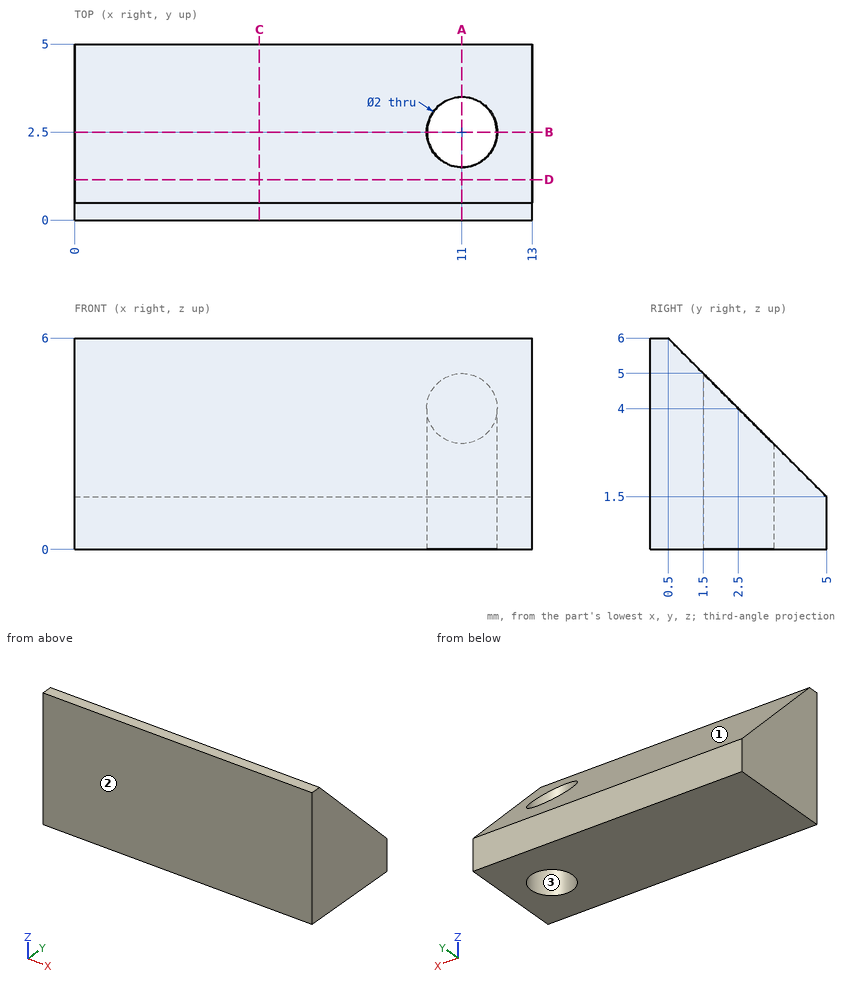
Geometry: see drawing. Coordinates: mm, zero at the bounding-box minimum. Coordinates: 2 decimals unless noted, no trailing zeros. Loops run counter-clockwise (first coordinate to the right, second up) from the corner with the lowest first, then second, coordinate; pieces in that order, holes last. Notation, with made-up numbers: (48.5, 27) - (107.5, 27) arc R18 cw to (107.5, 45) - close; hole circle Ø7 at (63.5, -1.5). An arc over 180 degrees is marked (long way). Answer in a Markdown table with one row per item.
(1) Cut plane A-A on x = 11. Output: boundary loops of the cut face in (y, z), plus the area to 3 significant figures.
Model answer:
| item | result |
|---|---|
| outline | (0, 0) - (1.5, 0) - (1.5, 5) - (0.5, 6) - (0, 6) - close; (3.5, 0) - (5, 0) - (5, 1.5) - (3.5, 3) - close |
| area | 11.9 mm² |
(2) Cut plane C-C on x = 5.25. Output: boundary loops of the cut face in (y, z).
Model answer:
| item | result |
|---|---|
| outline | (0, 0) - (5, 0) - (5, 1.5) - (0.5, 6) - (0, 6) - close |
(3) Cut plane B-B on y = 2.5. Output: boundary loops of the cut face in (x, z), plus the area to 3 significant figures.
Model answer:
| item | result |
|---|---|
| outline | (0, 0) - (10, 0) - (10, 4) - (0, 4) - close; (12, 0) - (13, 0) - (13, 4) - (12, 4) - close |
| area | 44.0 mm² |
(4) Mould query, pull axis Y, two halves, no side actions, for the marked faces 1, 2 and 3. Classes: pulls with the +Y half, pulls with the -Y half, needs draft (parallel to the pull), parting line crosses it, or undercut.
Model answer:
| item | result |
|---|---|
| face 1 | pulls with the +Y half |
| face 2 | pulls with the -Y half |
| face 3 | undercut |
(5) Pin query (flat end, axial travel): P1, Ø1, axis at y = 1.5, z = 1.5, coming from the -X side; P2, Ø3, axis at x = 9.5, y = 4, coming from the +Z side. Return the tip coordinate at first contact, or that it passes through.
Model answer:
| item | result |
|---|---|
| P1 | stops at x = 0 |
| P2 | stops at z = 4 |
(6) Material intervals for L1, parallel to X at y = 2.5, z = 2.15; L2, parallel to Y at x = 11, z = 2.05; L3, parallel to Y at x = 11, z = 3.05, sorted ascending. Write a range as from..to.
Model answer:
| item | result |
|---|---|
| L1 | x = 0..10, 12..13 |
| L2 | y = 0..1.5, 3.5..4.45 |
| L3 | y = 0..1.5 |
(7) Cut plane D-D on y = 1.15. Output: boundary loops of the cut face in (x, z), plus the area to 4 significant figures.
Model answer:
| item | result |
|---|---|
| outline | (0, 0) - (13, 0) - (13, 5.35) - (0, 5.35) - close |
| area | 69.55 mm² |
